from build123d import *

# Parameters (mm, degrees)
SKETCH1_W           = 55
SKETCH1_H           = 90.1
SKETCH1_R           = 2.05
BOSS_EXTRUDE2_DEPTH = 2
MIRROR1_OUTLINE_W   = 55
MIRROR1_OUTLINE_H   = 90.1
MIRROR1_OUTLINE_R   = 2.05
MIRROR1_DEPTH       = 2
SKETCH2_W           = 40.1
SKETCH2_H           = 5.1
CUT_EXTRUDE1_DEPTH  = 10
SKETCH3_R           = 1.1
SKETCH3_R_2         = 1.55
SKETCH3_R_3         = 1.390793096
SKETCH3_R_4         = 1.407266862
SKETCH3_R_5         = 1.402510713
SKETCH3_R_6         = 1.408268023
CUT_EXTRUDE2_DEPTH  = 10


# Read off the part's stored shape, not the designer's step: Mirror1
with BuildPart() as part:
    # Sketch1 → Boss-Extrude2 (new body)
    with BuildSketch(Plane(origin=(0, 0, 0), x_dir=(1, 0, 0), z_dir=(0, 1, 0))):
        with Locations((27.5, 45.05)):
            Rectangle(SKETCH1_W, SKETCH1_H)
        with Locations(Location((50, 77.1, 0), (0, 0, 270))):
            Circle(SKETCH1_R, mode=Mode.SUBTRACT)
        with Locations(Location((50, 60.1, 0), (0, 0, 270))):
            Circle(SKETCH1_R, mode=Mode.SUBTRACT)
        with Locations(Location((50, 35, 0), (0, 0, 270))):
            Circle(SKETCH1_R, mode=Mode.SUBTRACT)
    extrude(amount=BOSS_EXTRUDE2_DEPTH)

    # Mirror1 outline → Mirror1 (add)
    with BuildSketch(Plane(origin=(0, 0, 0), x_dir=(1, 0, 0), z_dir=(0, 1, 0))):
        with Locations((-27.5, 45.05)):
            Rectangle(MIRROR1_OUTLINE_W, MIRROR1_OUTLINE_H)
        with Locations((-50, 35)):
            Circle(MIRROR1_OUTLINE_R, mode=Mode.SUBTRACT)
        with Locations((-50, 60.1)):
            Circle(MIRROR1_OUTLINE_R, mode=Mode.SUBTRACT)
        with Locations((-50, 77.1)):
            Circle(MIRROR1_OUTLINE_R, mode=Mode.SUBTRACT)
    extrude(amount=MIRROR1_DEPTH)

    # Mirror2: part across plane


with BuildPart() as part_1:
    add(part.part)
    add(part.part.mirror(Plane(origin=(0, 2, 0), x_dir=(1, 0, 0), z_dir=(0, 0, -1))))

    # Sketch2 → Cut-Extrude1 (cut)
    with BuildSketch(Plane(origin=(0, 2, 0), x_dir=(1, 0, 0), z_dir=(0, 1, 0))):
        with Locations((0, 7.55)):
            Rectangle(SKETCH2_W, SKETCH2_H)
        with Locations((0, -7.55)):
            Rectangle(SKETCH2_W, SKETCH2_H)
    extrude(amount=-CUT_EXTRUDE1_DEPTH, mode=Mode.SUBTRACT)

    # Sketch3 → Cut-Extrude2 (cut)
    with BuildSketch(Plane(origin=(0, 2, 0), x_dir=(1, 0, 0), z_dir=(0, 1, 0))):
        with Locations(Location((-24.5, -77.1, 0), (0, 0, 270))):
            Circle(SKETCH3_R)
        with Locations(Location((24.5, -77.1, 0), (0, 0, 270))):
            Circle(SKETCH3_R)
        with Locations(Location((-38.5, -31.6, 0), (0, 0, 270))):
            Circle(SKETCH3_R)
        with Locations(Location((38.5, -31.6, 0), (0, 0, 270))):
            Circle(SKETCH3_R)
        with Locations(Location((23.55, 86.6, 0), (0, 0, 270))):
            Circle(SKETCH3_R_2)
        with Locations(Location((23.55, 23.55, 0), (0, 0, 270))):
            Circle(SKETCH3_R_2)
        with Locations(Location((-23.55, 86.6, 0), (0, 0, 270))):
            Circle(SKETCH3_R_2)
        with Locations(Location((-23.55, 23.55, 0), (0, 0, 270))):
            Circle(SKETCH3_R_2)
        with Locations(Location((0, -23.55, 0), (0, 0, 270))):
            Circle(SKETCH3_R_2)
        with Locations(Location((29.072459347, 78.586687626, 0), (0, 0, 270))):
            Circle(SKETCH3_R_3)
        with Locations(Location((29.255411637, 55.616498658, 0), (0, 0, 270))):
            Circle(SKETCH3_R_4)
        with Locations(Location((-28.941884451, 78.099990066, 0), (0, 0, 270))):
            Circle(SKETCH3_R_5)
        with Locations(Location((-28.741560934, 55.107175023, 0), (0, 0, 270))):
            Circle(SKETCH3_R_6)
    extrude(amount=-CUT_EXTRUDE2_DEPTH, mode=Mode.SUBTRACT)


solid = part_1.part
CAD build for the part. Positions are in the model's coordinates, mm. Coordinates: 2 decimals unless noted, no trailing zeros. Write each loop counter-clockwise with the first axis right and the second up, starting at its lowest first coordinate (ties: lowest second). Pieces come first, ordered by that corner, then holes. Notation, with made-up numbers: (22.25, 50.5) - (45.25, 50.5) arc R20 cw to (45.25, 68.5) - close; hole circle Ø4 at (55, 53). An arc over 180 degrees is marked (long way). Use a Markdown table: item, result. Add a question column.
Item 1: Drill centre lines: L1, parallel to Z at x = 4, y = 0.7; L2, parallel to X at y = 1.35, z = -60.1; L3, parallel to X at y = 0.65, z = -86.6. Where is each one in solid material? Low to high. Write a range as from..to.
Item 2: Mould opens along Z. For faces 1 (the face through (51.4, 1, 78.6)), 2 (the face through (-1, 0, 1)) say: pulls with the +Z half, pulls with the -Z half, needs draft (parallel to the pull), parting line crosses it, or undercut.
Item 3: Band-saw the part on A-A, the plane x = -50. Give the cut face in (y, z), and give its area (3 significant figures).
Item 4: Band-saw the part on C-C, the plane x = 17. Give the cut face in (y, z).
Item 5: Band-saw the part on D-D, the plane y = 1.6. Give the number of separate pieces and of enclosed holes in the cut face, and give its area (3 significant figures).
Item 6: Band-saw the part on B-B, the plane z = -35. Give the cut face in (x, y).
Numbers:
| question | item | result |
|---|---|---|
| 1 | L1 | -90.1..-10.1, -5..5, 10.1..90.1 |
| 1 | L2 | -55..-52.05, -47.95..47.95, 52.05..55 |
| 1 | L3 | -55..-25.1, -22..22, 25.1..55 |
| 2 | face 1 | undercut |
| 2 | face 2 | needs draft |
| 3 | outline | (0, -90.1) - (2, -90.1) - (2, -79.15) - (0, -79.15) - close; (0, -75.05) - (2, -75.05) - (2, -62.15) - (0, -62.15) - close; (0, -58.05) - (2, -58.05) - (2, -37.05) - (0, -37.05) - close; (0, -32.95) - (2, -32.95) - (2, 32.95) - (0, 32.95) - close; (0, 37.05) - (2, 37.05) - (2, 58.05) - (0, 58.05) - close; (0, 62.15) - (2, 62.15) - (2, 75.05) - (0, 75.05) - close; (0, 79.15) - (2, 79.15) - (2, 90.1) - (0, 90.1) - close |
| 3 | area | 311 mm2 |
| 4 | outline | (0, -90.1) - (2, -90.1) - (2, -10.1) - (0, -10.1) - close; (0, -5) - (2, -5) - (2, 5) - (0, 5) - close; (0, 10.1) - (2, 10.1) - (2, 90.1) - (0, 90.1) - close |
| 5 | separate pieces | 1 |
| 5 | enclosed holes | 27 |
| 5 | area | 19,200 mm2 |
| 6 | outline | (-55, 0) - (-52.05, 0) - (-52.05, 2) - (-55, 2) - close; (-47.95, 0) - (47.95, 0) - (47.95, 2) - (-47.95, 2) - close; (52.05, 0) - (55, 0) - (55, 2) - (52.05, 2) - close |
